from build123d import *

# Parameters (mm, degrees)
SKETCH1_R           = 16.539827403
BOSS_EXTRUDE1_DEPTH = 2.5
SKETCH3_R           = 9
BOSS_EXTRUDE3_DEPTH = 2.5
BOSS_EXTRUDE5_DEPTH = 14.25


with BuildPart() as part:
    # Sketch1 → Boss-Extrude1 (new, symmetric)
    with BuildSketch(Plane.XY):
        Circle(SKETCH1_R)
        with BuildLine():
            ThreePointArc((9, 0), (0, 9), (-9, 0))
            ThreePointArc((-9, 0), (0, -9), (9, 0))
        make_face(mode=Mode.SUBTRACT)
        with BuildLine():
            ThreePointArc((1.65, 12), (0, 13.65), (-1.65, 12))
            ThreePointArc((-1.65, 12), (0, 10.35), (1.65, 12))
        make_face(mode=Mode.SUBTRACT)
        with BuildLine():
            ThreePointArc((11.217304845, 4.571058084), (11.821246762, 6.825), (9.567304845, 7.428941916))
            ThreePointArc((9.567304845, 7.428941916), (8.963362929, 5.175), (11.217304845, 4.571058084))
        make_face(mode=Mode.SUBTRACT)
        with BuildLine():
            ThreePointArc((9.567304845, -7.428941916), (11.821246762, -6.825), (11.217304845, -4.571058084))
            ThreePointArc((11.217304845, -4.571058084), (8.963362929, -5.175), (9.567304845, -7.428941916))
        make_face(mode=Mode.SUBTRACT)
        with BuildLine():
            ThreePointArc((-1.65, -12), (0, -13.65), (1.65, -12))
            ThreePointArc((1.65, -12), (0, -10.35), (-1.65, -12))
        make_face(mode=Mode.SUBTRACT)
        with BuildLine():
            ThreePointArc((-11.217304845, -4.571058084), (-11.821246762, -6.825), (-9.567304845, -7.428941916))
            ThreePointArc((-9.567304845, -7.428941916), (-8.963362929, -5.175), (-11.217304845, -4.571058084))
        make_face(mode=Mode.SUBTRACT)
        with BuildLine():
            ThreePointArc((-9.567304845, 7.428941916), (-11.821246762, 6.825), (-11.217304845, 4.571058084))
            ThreePointArc((-11.217304845, 4.571058084), (-8.963362929, 5.175), (-9.567304845, 7.428941916))
        make_face(mode=Mode.SUBTRACT)
        with BuildLine():
            ThreePointArc((13.5, 0), (12, 1.5), (10.5, 0))
            ThreePointArc((10.5, 0), (12, -1.5), (13.5, 0))
        make_face(mode=Mode.SUBTRACT)
        with BuildLine():
            ThreePointArc((-10.5, 0), (-12, 1.5), (-13.5, 0))
            ThreePointArc((-13.5, 0), (-12, -1.5), (-10.5, 0))
        make_face(mode=Mode.SUBTRACT)
    extrude(amount=BOSS_EXTRUDE1_DEPTH, both=True)

    # Sketch3 → Boss-Extrude3 (add, symmetric)
    with BuildSketch(Plane.XY.offset(2.5)):
        Circle(SKETCH3_R)
    extrude(amount=BOSS_EXTRUDE3_DEPTH, both=True)

    # Sketch4 → Boss-Extrude5 (add)
    with BuildSketch(Plane.XY.offset(5)):
        with BuildLine():
            Line((-2, 4.582575695), (-2, 6))
            Line((-2, 6), (2, 6))
            Line((2, 6), (2, 4.582575695))
            ThreePointArc((2, 4.582575695), (0, -5), (-2, 4.582575695))
        make_face()
    extrude(amount=BOSS_EXTRUDE5_DEPTH)


solid = part.part
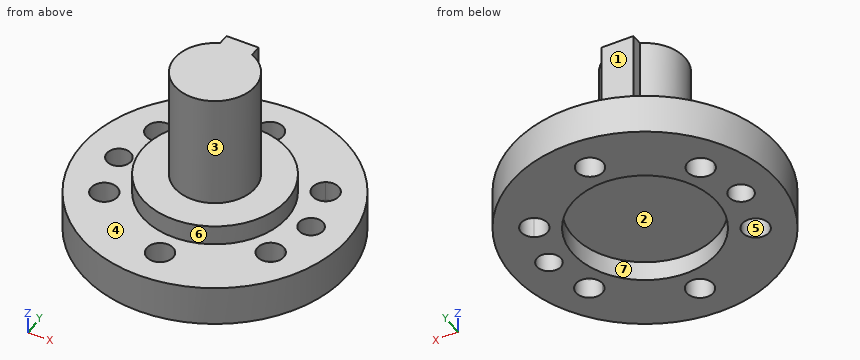
Build history of the part. All positions in model axes, mm. Face numbers are marked on the shaded views. A direction names the side the tool comes from. Round coordinates to 2 decimals unless told otherwise and drop trailing zeros. Loops run counter-clockwise (first coordinate to the right, second up) from the corner with the lowest first, then second, coordinate; pieces in that order, holes last. Notation, with made-up numbers: (22.25, -7) -> (46.25, -7) arc R18 cw to (46.25, -1) -> close; hole circle Ø6 at (-30.75, 19.25). An arc over 180 degrees is marked (long way). One line per item, written item: value. Start each with the question number.
Q1. Cut at A-A on y = 0. List the corners of the cut face in (x, z), plus the area to 3 significant figures.
Q2. Two-plate mould, pull along Y, no slides. Class the marked faces 1, 2, 3 and 4: released by +Y, released by -Y, zero draft, split by the parting line, or undercut.
Q3. Cut at B-B on x = 0. List the corners of the cut face in (y, z), plus the area to 3 significant figures.
Q4. Cut at C-C on y = -12. List the corners of the cut face in (x, z).
Q5. Drop flat-ended pins along their axis: pin 1 Ø1.5 at (y, z) = (-4.5, 6) entering from +X; pin 2 Ø2 at (x, y) = (-7, 10.5) entering from +Z; pin 3 Ø1.1 at (y, z) = (5.5, 14.5) entering from +X; pin 4 Ø1.8 at (x, y) = (-12, 0) entering from -Z. Give the stop position or say it passes through.
Q6. 3-axis set-ups, long thin cutter, end or side, ignore diameter. For the marked faces 5, 6 and 7: which of +Z, -Z, +X, -X, +Y, -Y reach the whole face in a straight line?
Q7. Probe line 1 along Y through (x, z) = (0, -1.05); line 2 along Y through (x, z) = (0, 1.75); line 3 along Z through (x, y) = (14, -3.5). List the from-to ranges inside material, lowest first.
Q8. Cut at D-D on z = 9.5. List the corners of the cut face in (x, y), plus the area to 3 significant figures.
Computed:
1. outline: (-16.54, -2.5) -> (-13.5, -2.5) -> (-13.5, 2.5) -> (-16.54, 2.5) -> close; (-10.5, -2.5) -> (-9, -2.5) -> (-9, 0) -> (9, 0) -> (9, -2.5) -> (10.5, -2.5) -> (10.5, 2.5) -> (9, 2.5) -> (9, 5) -> (5, 5) -> (5, 19.25) -> (-5, 19.25) -> (-5, 5) -> (-9, 5) -> (-9, 2.5) -> (-10.5, 2.5) -> close; (13.5, -2.5) -> (16.54, -2.5) -> (16.54, 2.5) -> (13.5, 2.5) -> close
1. area: 278 mm²
2. face 1: released by +Y
2. face 2: undercut
2. face 3: split by the parting line
2. face 4: zero draft
3. outline: (-16.54, -2.5) -> (-13.65, -2.5) -> (-13.65, 2.5) -> (-16.54, 2.5) -> close; (-10.35, -2.5) -> (-9, -2.5) -> (-9, 0) -> (9, 0) -> (9, -2.5) -> (10.35, -2.5) -> (10.35, 2.5) -> (9, 2.5) -> (9, 5) -> (6, 5) -> (6, 19.25) -> (-5, 19.25) -> (-5, 5) -> (-9, 5) -> (-9, 2.5) -> (-10.35, 2.5) -> close; (13.65, -2.5) -> (16.54, -2.5) -> (16.54, 2.5) -> (13.65, 2.5) -> close
3. area: 289 mm²
4. outline: (-11.38, -2.5) -> (-1.65, -2.5) -> (-1.65, 2.5) -> (-11.38, 2.5) -> close; (1.65, -2.5) -> (11.38, -2.5) -> (11.38, 2.5) -> (1.65, 2.5) -> close
5. pin 1: x = 3.31
5. pin 2: z = 2.5
5. pin 3: x = 2
5. pin 4: through
6. face 5: +Z, -Z
6. face 6: +Z
6. face 7: -Z
7. line 1: -16.54 to -13.65, -10.35 to -9, 9 to 10.35, 13.65 to 16.54
7. line 2: -16.54 to -13.65, -10.35 to 10.35, 13.65 to 16.54
7. line 3: -2.5 to 2.5
8. outline: (-2, 4.58) arc R5 ccw (long way) to (2, 4.58) -> (2, 6) -> (-2, 6) -> close
8. area: 83.1 mm²
